from build123d import *

# Parameters (mm, degrees)
F0_R     = 9.5
F1_DEPTH = 11
F2_R     = 9
F3_DEPTH = 30
F5_R     = 11
F6_DEPTH = 5.5
F7_R     = 5.5
F8_DEPTH = 38.19265


with BuildPart() as f1:
    # F0 (on Right) → F1 (new body, symmetric)
    with BuildSketch(Plane.YZ):
        Circle(F0_R)
    extrude(amount=F1_DEPTH, both=True)

    # F2 (on Top) → F3 (join)
    with BuildSketch(Plane.XY):
        Circle(F2_R)
    extrude(amount=F3_DEPTH)

    # F5 (on Right) → F6 (join, symmetric)
    with BuildSketch(Plane.YZ):
        Circle(F5_R)
    extrude(amount=F6_DEPTH, both=True)

    # F7 (on offset) → F8 (cut, symmetric)
    with BuildSketch(Plane.YZ.offset(13)):
        Circle(F7_R)
    extrude(amount=F8_DEPTH, both=True, mode=Mode.SUBTRACT)


solid = f1.part
Here's how the part is built. I have some questions about the finished solid (model axes, mm). A direction names the side the tool comes from. Coordinates: 2 decimals unless noted, no trailing zeros. Loops run counter-clockwise (first coordinate to the right, second up) from the corner with the lowest first, then second, coordinate; pieces in that order, holes last.
1. Imagine slicing it at B-B, the plane y = 0. Please give me the cut outline in (x, z), and give its area (4 significant figures).
2. Imagine slicing it at A-A, the plane z = 0. Please give me the cut outline in (x, y), and give its area (3 significant figures).
3. Imagine slicing it at D-D, the plane y = -8.25. Please give me the cut outline in (x, z).
4. For P1, Ø6.5, axis at y = 0, z = 0, coming from the -X side; P2, Ø1.5, axis at y = 1.5, z = 20.5, coming from the -X side; P3, Ø1, axis at x = -8.5, z = -6, coming from the +Y side; P4, Ø10, axis at x = -2, y = -0.5, coming from the -Z side, each with a flat end and sliding along its axis, tell me the tip position at first contact or that it passes through.
5. I need wall thicknesses on L1, parallel to Z at x = -1, y = 0; L2, parallel to Z at x = -3, y = 3.5; L3, parallel to X at y = 10, z = -2. Which ranges of each line are inside material? Lowest first, please.
6. Imagine slicing it at C-C, the plane x = 1.25. Please give me the cut outline in (y, z), and give its area (3 significant figures).
7. For faces 1 (the flat face through (5.5, 0, -10)), 2 (the flat face through (0, 0, 30)), 3 (the cylindrical face through (-8.211, -2.059, -9.274)), which set-ups out of +Z, -Z, +X, -X, +Y, -Y let a thin tool reach every point of the face, with its end or its side?
8. If we mould it in two halves opening along Y, with no side actions, what happens to faces 4 (the cylindrical face through (-6.633, 6.083, 17.976)), 5 (the flat face through (11, 4, -4)), 6 (the cylindrical face through (0.15, -1.19, -5.37))? For each: pulls with the +Y half, pulls with the -Y half, needs draft (parallel to the pull), parting line crosses it, or undercut.
Taken from the geometry:
1. outline: (-11, -9.5) - (-5.5, -9.5) - (-5.5, -11) - (5.5, -11) - (5.5, -9.5) - (11, -9.5) - (11, -5.5) - (-11, -5.5) - close; (-11, 5.5) - (11, 5.5) - (11, 9.5) - (9, 9.5) - (9, 30) - (-9, 30) - (-9, 9.5) - (-11, 9.5) - close
1. area: 561.5 mm2
2. outline: (-11, -9.5) - (-5.5, -9.5) - (-5.5, -11) - (5.5, -11) - (5.5, -9.5) - (11, -9.5) - (11, -5.5) - (-11, -5.5) - close; (-11, 5.5) - (11, 5.5) - (11, 9.5) - (5.5, 9.5) - (5.5, 11) - (-5.5, 11) - (-5.5, 9.5) - (-11, 9.5) - close
2. area: 209 mm2
3. outline: (-11, -4.71) - (-5.5, -4.71) - (-5.5, -7.28) - (5.5, -7.28) - (5.5, -4.71) - (11, -4.71) - (11, 4.71) - (5.5, 4.71) - (5.5, 7.28) - (3.6, 7.28) - (3.6, 30) - (-3.6, 30) - (-3.6, 7.28) - (-5.5, 7.28) - (-5.5, 4.71) - (-11, 4.71) - close
4. P1: passes through
4. P2: stops at x = -8.97
4. P3: stops at y = 7.75
4. P4: stops at z = -11
5. L1: z = -11 to -5.5, 5.5 to 30
5. L2: z = -10.43 to -4.24, 4.24 to 30
5. L3: x = -5.5 to 5.5
6. outline: (-8.91, 6.45) arc R11 ccw (long way) to (8.91, 6.45) - (8.91, 30) - (-8.91, 30) - close; hole circle Ø11 at (0, 0)
6. area: 648 mm2
7. face 1: +X
7. face 2: +Z, +X, -X, +Y, -Y
7. face 3: -X
8. face 4: parting line crosses it
8. face 5: needs draft
8. face 6: undercut
